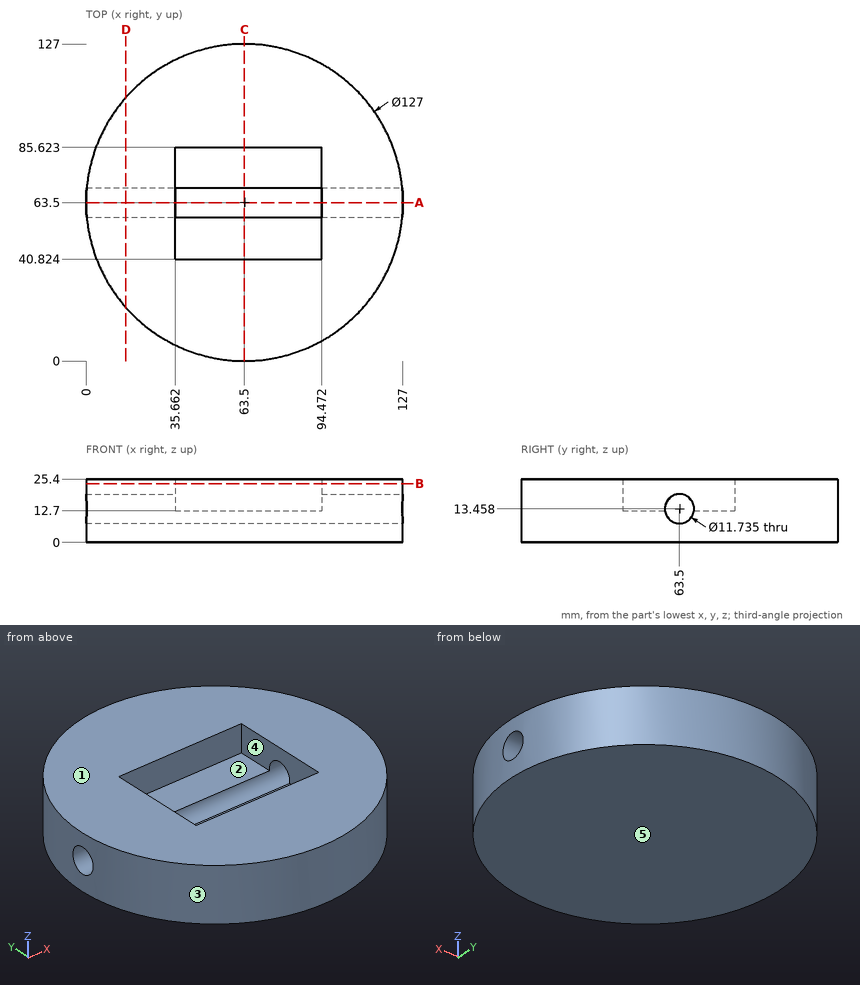
Study the drawing (mm; zero at the part's minimum x, y, z) and answer. A direction names the side the tool comes from. Give positions to 0.01 mm unless a question says otherwise; leave off trailing zeros. Order: outer loops, then holes, each group sorted by start corner. A loop starts at its lowest first (then second) coordinate and runs counter-clockwise, first axis right, second up. Notation, with made-up numbers: (42, 84.5) - (73, 84.5) arc R28 cw to (73, 117.5) - close; hole circle Ø4 at (-26.5, 74). An arc over 180 degrees is marked (long way). Use one line per item in the form item = value. Start each with the question number.
(1) A cutting plane is placed at C-C, the plane x = 63.5. Write down the section's boundary in (y, z) (1 decimal), then the cut area to 3 significant figures.
(2) A cutting plane is placed at D-D, the plane x = 16. Write down the section's boundary in (y, z) (1 decimal), then the cut area to 3 significant figures.
(3) A cutting plane is placed at B-B, the plane z = 23.5. Write down the section's boundary in (x, y) (1 decimal).
(4) Consider line 1 (Z direction, x = 69.5, y = 63.5); line 2 (Z direction, x = 64.5, y = 76); line 3 (Y direction, x = 70.5, z = 10.5). Determine where each line is inside the solid, lowest interval first. Write a range as from..to.
(5) The mould has two halves that part along Y. Classify the marked faces 3, 4 and 5: released by +Y, released by -Y, zero draft, split by the parting line, or undercut.
(6) A cutting plane is placed at A-A, the plane y = 63.5. Write down the section's boundary in (x, z) (1 decimal), then the cut area to 3 significant figures.
(7) Flat-ended cylindrical pins translate along their axes: pin 1 Ø10 at (x, z) = (92, 9.5) entering from +Y; pin 2 Ø6 at (y, z) = (61.5, 9) entering from +X; pin 3 Ø4 at (y, z) = (79, 9.5) entering from +X; pin 4 Ø12 at (y, z) = (72, 16) entering from -X. Find the tip coordinate at first contact, or state that the pin passes through.
(8) For the marked faces 1 and 2, determine the directions among +Z, -Z, +X, -X, +Y, -Y from which every point of the face is accessible in a straight line to the end or side of a thin tool.
Ans:
q1.outline = (0, 0) - (127, 0) - (127, 25.4) - (85.6, 25.4) - (85.6, 12.7) - (69.3, 12.7) arc R5.9 cw to (57.7, 12.7) - (40.8, 12.7) - (40.8, 25.4) - (0, 25.4) - close
q1.area = 2,610 mm^2
q2.outline = (21.4, 0) - (105.6, 0) - (105.6, 25.4) - (21.4, 25.4) - close; hole circle Ø11.7 at (63.5, 13.5)
q2.area = 2,030 mm^2
q3.outline = circle Ø127 at (63.5, 63.5); hole (35.7, 40.8) - (94.5, 40.8) - (94.5, 85.6) - (35.7, 85.6) - close
q4.line_1 = 0..7.59
q4.line_2 = 0..12.7
q4.line_3 = 0.39..58.43, 68.57..126.61
q5.face_3 = split by the parting line
q5.face_4 = undercut
q5.face_5 = zero draft
q6.outline = (0, 0) - (127, 0) - (127, 7.6) - (0, 7.6) - close; (0, 19.3) - (35.7, 19.3) - (35.7, 25.4) - (0, 25.4) - close; (94.5, 19.3) - (127, 19.3) - (127, 25.4) - (94.5, 25.4) - close
q6.area = 1,380 mm^2
q7.pin_1 = 122.49
q7.pin_2 = 127
q7.pin_3 = 125.55
q7.pin_4 = 0.07
q8.face_1 = +Z, +X, -X, +Y, -Y
q8.face_2 = +Z
